For this review, use the dimensioned drawing (mm, ordinates from the lowest corner) and the shaded views. A direction names the side the tool comes from. Round coordinates to 2 decimals unless told otherwise and drop trailing zeros. Order: outer loops, then holes, each group sorted by start corner. A loop starts at its lowest first (then second) coordinate and runs counter-clockwise, first axis right, second up. Notation, with made-up numbers: (41.25, -8.75) - (70.25, -8.75) arc R24 cw to (70.25, 16.25) - close; hole circle Ø7 at (82.5, 51). An arc over 180 degrees is marked (long way). Write item = value, one per line.
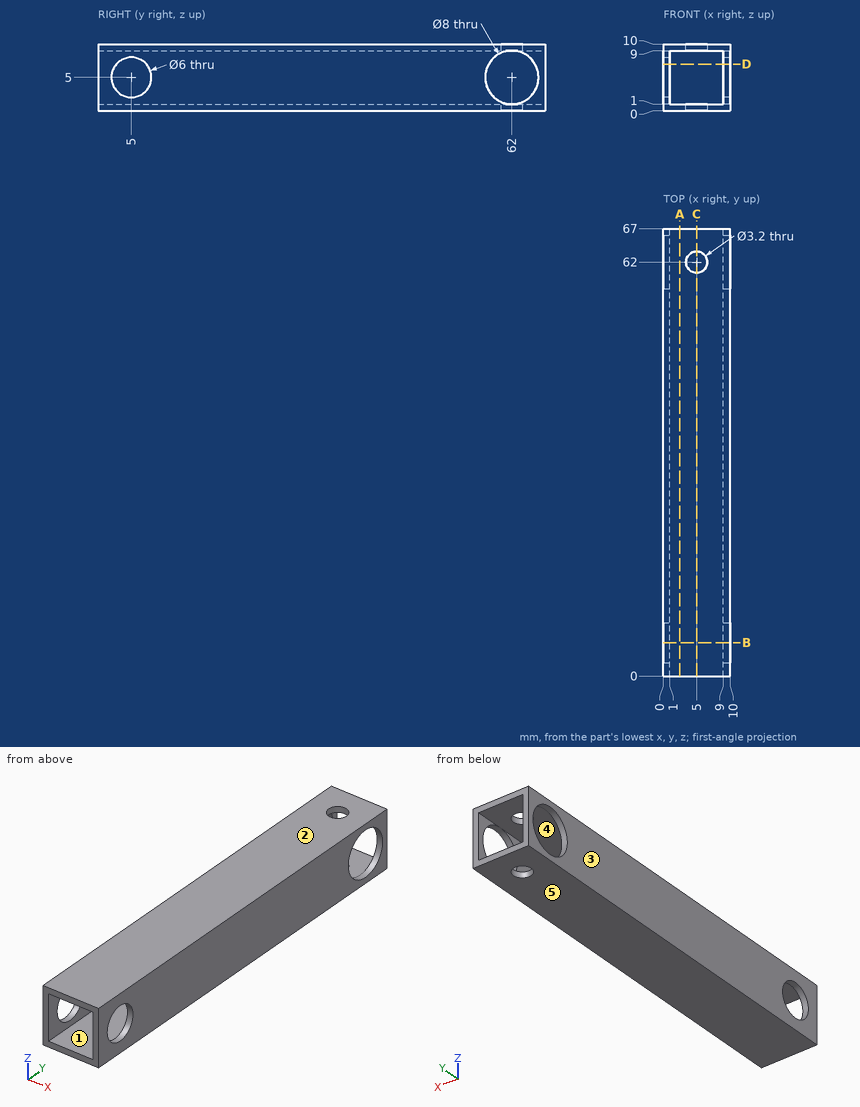
1) We need section B-B on y = 5. Write out the cut boundary in (x, z).
Findings:
outline = (0, 0) - (10, 0) - (10, 2) - (9, 2) - (9, 1) - (1, 1) - (1, 2) - (0, 2) - close; (0, 8) - (1, 8) - (1, 9) - (9, 9) - (9, 8) - (10, 8) - (10, 10) - (0, 10) - close
2) For the marked faces 1 and 2, list the 3-axis set-ups (+Z, -Z, +X, -X, +Y, -Y) from which the entire face can be reached by the end or side of a thin tool; tool diameter is ignored.
Findings:
face_1 = +Y, -Y
face_2 = +Z, +X, -X, +Y, -Y
3) To check wall thickness, follow L1, parallel to Y at x = 9.75, z = 5; L2, parallel to X at y = 31.5, z = 6.5. State the ranges of each line that lie inside material, in increasing order. Write a range as from..to.
Findings:
L1 = 0..2, 8..58, 66..67
L2 = 0..1, 9..10
4) We need section D-D on z = 7. Write out the cut boundary in (x, y), and give its area (3 significant figures).
Findings:
outline = (0, 0) - (1, 0) - (1, 2.76) - (0, 2.76) - close; (0, 7.24) - (1, 7.24) - (1, 58.54) - (0, 58.54) - close; (0, 65.46) - (1, 65.46) - (1, 67) - (0, 67) - close; (9, 0) - (10, 0) - (10, 2.76) - (9, 2.76) - close; (9, 7.24) - (10, 7.24) - (10, 58.54) - (9, 58.54) - close; (9, 65.46) - (10, 65.46) - (10, 67) - (9, 67) - close
area = 111 mm^2
5) We need section C-C on x = 5. Write out the cut boundary in (y, z).
Findings:
outline = (0, 0) - (60.4, 0) - (60.4, 1) - (0, 1) - close; (0, 9) - (60.4, 9) - (60.4, 10) - (0, 10) - close; (63.6, 0) - (67, 0) - (67, 1) - (63.6, 1) - close; (63.6, 9) - (67, 9) - (67, 10) - (63.6, 10) - close
6) The part is to be moulded in two halves that separate along Z. For the marked faces 3, 4 and 5, say which applies: released by +Z, released by -Z, zero draft, split by the parting line, or undercut.
Findings:
face_3 = zero draft
face_4 = undercut
face_5 = released by -Z
7) We need section A-A on x = 2.5. Write out the cut boundary in (y, z).
Findings:
outline = (0, 0) - (67, 0) - (67, 1) - (0, 1) - close; (0, 9) - (67, 9) - (67, 10) - (0, 10) - close
